The listing builds one solid part. Answer for the finished solid, in the listing's coordinates (mm). Give positions to 0.01 mm unless a question says otherwise; leave off trailing zeros. Write each loop counter-clockwise with the first axis right and the second up, starting at its lowest first coordinate (ties: lowest second). Pieces come first, ordered by that corner, then holes.
Autodesk Inventor part; units mm, degrees
ref_plane "Work Plane1" through (0, 0, 3.175) normal (0, 0, 1) x (1, 0, 0)
ref_plane "YZ Plane" through (0, 0, 0) normal (1, 0, 0) x (0, 1, 0)
ref_plane "XZ Plane" through (0, 0, 0) normal (0, 1, 0) x (-1, 0, 0)
sketch "Sketch1" plane through (0, 0, 0) normal (0, 1, 0) x (-1, 0, 0)
  circle A0 centre (0, 0) radius 3.175
  circle A1 centre (0, 0) radius 1.5
  dimension "d0" = 6.35
  dimension "d1" = 3
extrude "Extrusion1" add sketch "Sketch1" against normal blind 7.5 contours A0 | A1
hole "Hole1" at (0, 0, 0) direction (0, -1, 0) diameter 3.2004 depth 1.5 tip angle 118
ref_plane "Work Plane1" through (0, 0, 3.175) normal (0, 0, 1) x (1, 0, 0)
sketch "Sketch2" plane through (0, 0, 3.175) normal (0, 0, 1) x (1, 0, 0)
  line L0 (-3.175, -7.5) -> (3.175, -7.5)
  line L1 (3.175, 0) -> (-3.175, 0)
  line L2 (-3.175, 0) -> (-3.175, -7.5)
  line L3 (-3.175, -2) -> (3.175, -2) construction
  circle A0 centre (0, -4.75) radius 1.5
  dimension "d11" = 2
  dimension "d12" = 3
  dimension "d13" = 2.75
  dimension "d14" = 3.175
hole "Hole2" at (0, -4.75, 3.175) direction (0, 0, -1) diameter 2.459 end through all
properties part number "Bearing Nut" material "Aluminum 6061"
Item 1: Consider probe 1 along X at (y, z) = (-5, 2.5); probe 2 along Y at (x, z) = (0.5, 0.75); probe 3 along Y at (x, z) = (0.25, -3). Determine where each line is inside the solid, lowest interval first.
Conclusion:
probe 1: x = -1.96 to -1.2, 1.2 to 1.96
probe 2: y = -7.5 to -5.87, -3.63 to -1.92
probe 3: y = -7.5 to -5.95, -3.55 to 0
Item 2: A cutting plane is placed at A-A, the plane y = -0.25. Give the vertices of the cut face in (x, z) (3 decimals), plus the area to 3 significant figures.
Conclusion:
outline: circle Ø6.35 at (0, 0); hole circle Ø3.2 at (0, 0)
area: 23.6 mm2
Item 3: A cutting plane is placed at B-B, the plane y = -2.75. Give the vertices of the cut face in (x, z) (3 decimals).
Conclusion:
outline: circle Ø6.35 at (0, 0)
Item 4: Determine the mould class of faces 1 (the face through (0.974, -0.76, -1.27)), 2 (the face through (0, -7.5, 0)), 3 (the face through (-1.5, -3.7, -2.8)), 4 (the face through (-0.271, -2.295, -0.06)) for opening direction Z: pulls with the +Z half, pulls with the -Z half, needs draft (parallel to the pull), parting line crosses it, or undercut.
Conclusion:
face 1: undercut
face 2: needs draft
face 3: parting line crosses it
face 4: undercut
Item 5: Each of these flat-tipped pins is pushed along its axis until it touches: P1, Ø3, axis at x = 0.5, y = -1.5, coming from the -Z side (3 decimals); P2, Ø1.5, axis at x = 2, y = -3, coming from the -Z side; P3, Ø1.5, axis at y = -3.5, z = -2.5, coming from the -X side. Where does it stop, or does it pass through?
Conclusion:
P1: stops at z = -3.175
P2: stops at z = -2.92
P3: stops at x = -2.65
Item 6: A cutting plane is placed at D-D, the plane x = -2.5. Give the vertices of the cut face in (y, z), plus the area to 3 significant figures.
Conclusion:
outline: (-7.5, -1.96) - (0, -1.96) - (0, 1.96) - (-7.5, 1.96) - close
area: 29.4 mm2
